Input: dimensioned drawing with shaded views. Units: mm. Origin: part minimum x, y, z. A direction names the side the tool comes from. Round coordinates to 2 decimals unless told otherwise and drop trailing zeros. Loops run counter-clockwise (first coordinate to the right, second up) from the corner with the lowest first, then second, coordinate; pieces in that order, holes last.
1) Section C-C, the plane z = 10. Return loops of the section in (x, y), and give its area (3 significant figures).
2) First-contact query: pin 1 (1.1 mm diameter, centred on x = 29.5, y = 4, fed in from -Z); pin 2 (2.5 mm diameter, centred on x = 27.5, y = 3, fed in from -Z). Flat tips, straight axial feed; report the tip coordinate or a pass-through.
3) Section A-A, the plane x = 13.75. Return loops of the section in (y, z).
4) Section B-B, the plane y = 5.5. Return loops of the section in (x, z).
5) Access query for the marked faces 5, 6 and 7. Directions: +Z, -Z, +X, -X, +Y, -Y. A direction counts if a zero-diameter tool reaches every point of the face in a straight line with its end or side. Return the directions, or none.
6) Section D-D, the plane z = 5.5. Return loops of the section in (x, y), and give its area (3 significant figures).
7) Draft query along X for the marked faces 1, 2, 3 and 4. Return one class per face: pulls with the +X half, pulls with the -X half, needs draft (parallel to the pull), parting line crosses it, or undercut.
8) Ray query, line 1 along Z through (x, y) = (4.25, 4.75); line 2 along X through (y, z) = (2.5, 8); line 3 along Z through (x, y) = (13.75, 3.5). Return the intervals inside material, ascending.
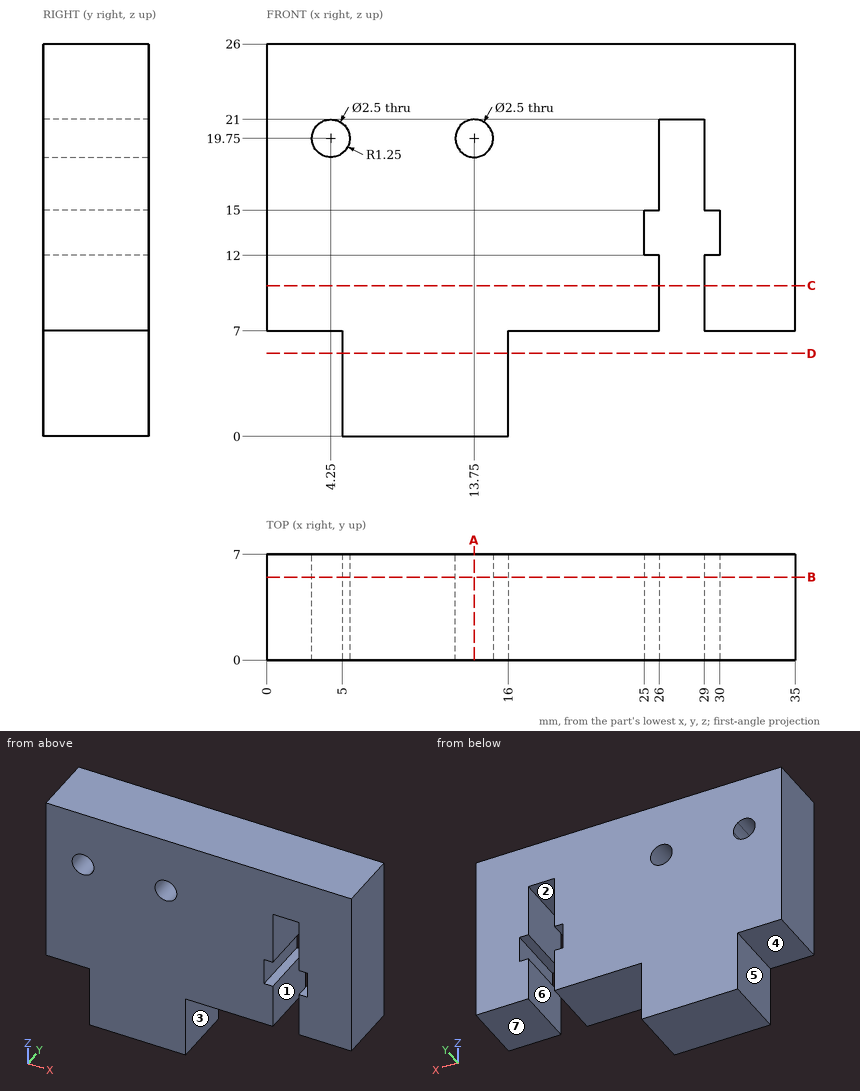
Final values:
1. outline: (0, 0) - (26, 0) - (26, 7) - (0, 7) - close; (29, 0) - (35, 0) - (35, 7) - (29, 7) - close
1. area: 224 mm2
2. pin 1: stops at z = 7
2. pin 2: stops at z = 21
3. outline: (0, 0) - (7, 0) - (7, 18.5) - (0, 18.5) - close; (0, 21) - (7, 21) - (7, 26) - (0, 26) - close
4. outline: (0, 7) - (5, 7) - (5, 0) - (16, 0) - (16, 7) - (26, 7) - (26, 12) - (25, 12) - (25, 15) - (26, 15) - (26, 21) - (29, 21) - (29, 15) - (30, 15) - (30, 12) - (29, 12) - (29, 7) - (35, 7) - (35, 26) - (0, 26) - close; hole circle Ø2.5 at (4.25, 19.75); hole circle Ø2.5 at (13.75, 19.75)
5. face 5: -Z, -X, +Y, -Y
5. face 6: -Z, +Y, -Y
5. face 7: -Z, +X, +Y, -Y
6. outline: (5, 0) - (16, 0) - (16, 7) - (5, 7) - close
6. area: 77.0 mm2
7. face 1: undercut
7. face 2: undercut
7. face 3: pulls with the +X half
7. face 4: needs draft
8. line 1: z = 7 to 18.5, 21 to 26
8. line 2: x = 0 to 26, 29 to 35
8. line 3: z = 0 to 18.5, 21 to 26
